The model under review builds one solid part; all positions refer to its coordinate system, in mm. Face numbers are marked on the shaded views. A direction names the side the tool comes from. Round coordinates to 2 decimals unless told otherwise and drop trailing zeros. Order: outer loops, then holes, each group sorted by start corner. A loop starts at its lowest first (then second) coordinate and runs counter-clockwise, first axis right, second up. Notation, with made-up numbers: (7, 79.5) -> (42, 79.5) arc R20 cw to (42, 95.5) -> close; hole circle Ø2 at (13, -21). An arc over 180 degrees is marked (long way). Use a Markdown table: item, result. Add a question column.
```python
from build123d import *

# Parameters (mm, degrees)
SKETCH3_W           = 1
SKETCH3_H           = 0.5
BOSS_EXTRUDE1_DEPTH = 2
BOSS_EXTRUDE2_START = 1.5
SKETCH3_3_W         = 1
SKETCH3_3_H         = 0.5
BOSS_EXTRUDE2_DEPTH = 0.5
SKETCH5_W           = 1
SKETCH5_H           = 0.5
BOSS_EXTRUDE3_DEPTH = 2
BOSS_EXTRUDE4_START = 1.5
SKETCH5_3_W         = 1
SKETCH5_3_H         = 0.5
BOSS_EXTRUDE4_DEPTH = 0.5


with BuildPart() as part:
    # Sweep1: sweep along a path in Sketch2
    with BuildLine(Plane.YZ) as sweep1_path:
        Line((0, 0), (0, 5.289768345))
        ThreePointArc((0, 5.289768345), (-1.636519098, 14.186271038), (-6.331820813, 21.918030005))
        Line((-6.331820813, 21.918030005), (-33.668179187, 52.60795099))
        ThreePointArc((-33.668179187, 52.60795099), (-38.363480902, 60.339709958), (-40, 69.23621265))
        Line((-40, 69.23621265), (-40, 80))
    # Sketch1 → Sweep1 (sweep)
    with BuildSketch(Plane.XY):
        with BuildLine():
            ThreePointArc((3.333333333, 5.5), (3.833333333, 6), (4.333333333, 5.5))
            Line((4.333333333, 5.5), (4.333333333, 0))
            Line((4.333333333, 0), (-4.333333333, 0))
            Line((-4.333333333, 0), (-4.333333333, 5.5))
            ThreePointArc((-4.333333333, 5.5), (-3.833333333, 6), (-3.333333333, 5.5))
            Line((-3.333333333, 5.5), (-3.333333333, 0.5))
            Line((-3.333333333, 0.5), (3.333333333, 0.5))
            Line((3.333333333, 0.5), (3.333333333, 5.5))
        make_face()
    sweep(path=sweep1_path.line)

    # Sketch3 → Boss-Extrude1 (add)
    with BuildSketch(Plane.XY.offset(80)):
        with Locations((-3.833333333, -39.25)):
            Rectangle(SKETCH3_W, SKETCH3_H)
        with Locations((3.833333333, -39.25)):
            Rectangle(SKETCH3_W, SKETCH3_H)
    extrude(amount=BOSS_EXTRUDE1_DEPTH)

    # Sketch3<3> → Boss-Extrude2 (add)
    with BuildSketch(Plane.XY.offset(80).offset(BOSS_EXTRUDE2_START)):
        with Locations((-3.833333333, -39.75)):
            Rectangle(SKETCH3_3_W, SKETCH3_3_H)
        with Locations((3.833333333, -39.75)):
            Rectangle(SKETCH3_3_W, SKETCH3_3_H)
    extrude(amount=BOSS_EXTRUDE2_DEPTH)

    # Sketch5 → Boss-Extrude3 (add)
    with BuildSketch(Plane(origin=(0, 0, 0), x_dir=(-1, 0, 0), z_dir=(0, 0, -1))):
        with Locations((3.833333333, 0.75)):
            Rectangle(SKETCH5_W, SKETCH5_H)
        with Locations((-3.833333333, 0.75)):
            Rectangle(SKETCH5_W, SKETCH5_H)
    extrude(amount=BOSS_EXTRUDE3_DEPTH)

    # Sketch5<3> → Boss-Extrude4 (add)
    with BuildSketch(Plane(origin=(0, 0, 0), x_dir=(-1, 0, 0), z_dir=(0, 0, -1)).offset(BOSS_EXTRUDE4_START)):
        with Locations((-3.833333333, 0.25)):
            Rectangle(SKETCH5_3_W, SKETCH5_3_H)
        with Locations((3.833333333, 0.25)):
            Rectangle(SKETCH5_3_W, SKETCH5_3_H)
    extrude(amount=BOSS_EXTRUDE4_DEPTH)


solid = part.part
```
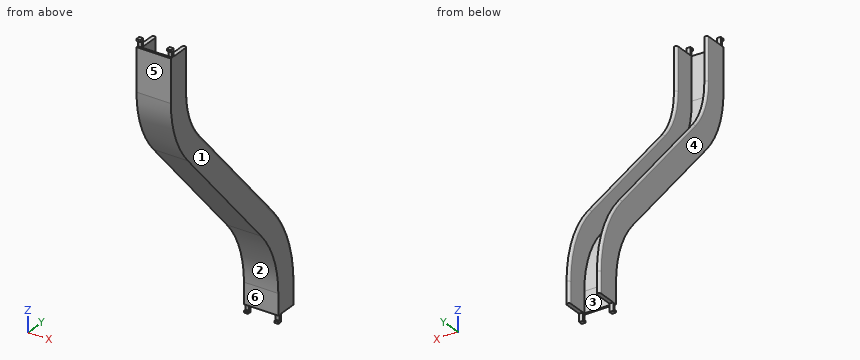
Q1. For the marked faces 5 and 6, list the 3-axis set-ups (+Z, -Z, +X, -X, +Y, -Y) from which the entire face can be reached by the end or side of a thin tool; tool diameter is ignored.
Q2. Draft analysis for pull direction X (two halves, no side actions). For the marked faces 1, 2, 3 and 4, state which applies: released by +X, released by -X, zero draft, split by the parting line, or undercut.
Q3. Add section A-A, the plane x = -1. Give the boundary of the cut face in (y, z), then the cut area to 3 significant figures.
Q4. To check wall thickness, follow line 1 along Y through (x, z) = (0.5, 78); line 2 along Z through (x, y) = (-1.25, -20.5); line 3 along Y through (x, z) = (-2.25, 24.5). State the ranges of each line that lie inside material, in increasing order.
Q5. For pin 1 (0.8 mm diameter, centred on x = 4, z = 81, fed in from -Y); pin 2 (2 mm diameter, centred on x = -3.5, y = -26, fed in from -Z); pin 3 (2 mm diameter, centred on x = -1, z = 77.5, fed in from +Y), all flat-tipped, find the tip position at first contact; note any pin that passes through.
Return value:
| question | item | result |
|---|---|---|
| 1 | face 5 | +Z, -Z, +X, -X, -Y |
| 1 | face 6 | -Z, +X, -X, -Y |
| 2 | face 1 | released by +X |
| 2 | face 2 | zero draft |
| 2 | face 3 | undercut |
| 2 | face 4 | released by -X |
| 3 | outline | (-40, 69.24) arc R25 ccw to (-33.67, 52.61) -> (-6.33, 21.92) arc R25 cw to (0, 5.29) -> (0, 0) -> (0.5, 0) -> (0.5, 5.29) arc R25.5 ccw to (-5.96, 22.25) -> (-33.29, 52.94) arc R24.5 cw to (-39.5, 69.24) -> (-39.5, 80) -> (-40, 80) -> close |
| 3 | area | 46.8 mm² |
| 4 | line 1 | -40 to -39.5 |
| 4 | line 2 | 37.82 to 38.58 |
| 4 | line 3 | -8.63 to -7.96 |
| 5 | pin 1 | y = -39.5 |
| 5 | pin 2 | z = 42.88 |
| 5 | pin 3 | y = -39.5 |
